Print and shaded views of the part. All mm, measured from the part's lowest x, y and z. Round coordinates to 2 decimals unless told otherwise and drop trailing zeros. Write each loop counter-clockwise with the first axis right and the second up, starting at its lowest first coordinate (ties: lowest second). Pieces come first, ordered by that corner, then holes. Notation, with made-up numbers: (58.5, 55.5) - (73.5, 55.5) arc R29 ccw to (73.5, 93.5) - close; hole circle Ø6 at (81, 75.25). An arc over 180 degrees is marked (long way). Put each result on its own line as item: value. Start each with the question number.
Item 1: Cut at A-A (x = 15.24). Give the cut face in (y, z) (1 decimal).
Item 2: Pin check, flat tips, straight feed: pin 1 Ø5 at (y, z) = (7.5, 146) entering from +X; pin 2 Ø1.5 at (x, z) = (104, 76.5) entering from +Y (3 decimals); pin 3 Ø3.5 at (x, y) = (124.26, 9.325) entering from -Z; pin 4 Ø5.5 at (x, y) = (69.75, 9.325) entering from -Z. Stop position of each tip, or through.
Item 3: Cut at B-B (z = 50). Give the cut face in (x, y) (1 decimal), and give its area (3 significant figures).
Item 4: Cut at C-C (x = 51.5). Give the cut face in (y, z) (1 decimal).
Item 5: Drill centre lines: line 1 (X direction, y = 9, z = 141); line 2 (Y direction, x = 57.5, z = 35.5) (1 decimal); line 3 (X direction, y = 4.25, z = 141.5). Where is each one in solid material? Low to high. Write a range as from..to.
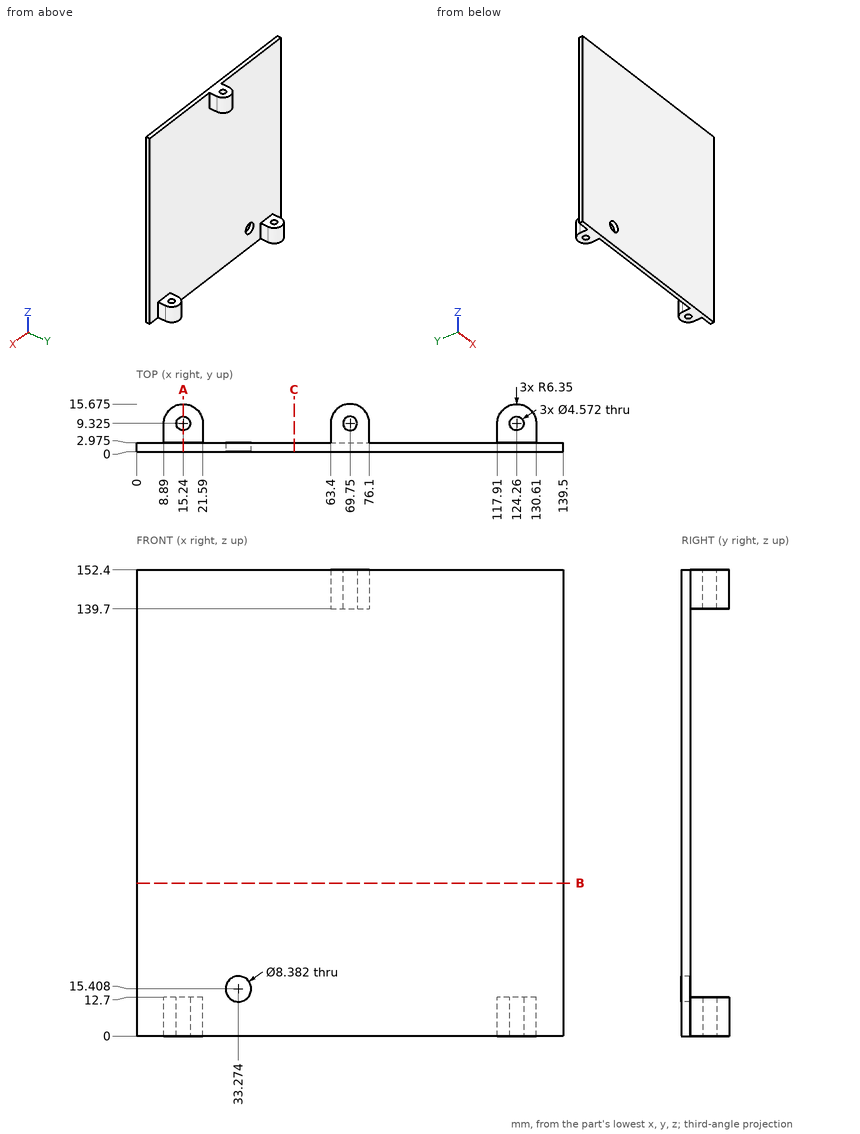
Output values:
1. outline: (0, 0) - (7, 0) - (7, 12.7) - (3, 12.7) - (3, 152.4) - (0, 152.4) - close; (11.6, 0) - (15.7, 0) - (15.7, 12.7) - (11.6, 12.7) - close
2. pin 1: x = 76.1
2. pin 2: y = 2.975
2. pin 3: through
2. pin 4: z = 139.7
3. outline: (0, 0) - (139.5, 0) - (139.5, 3) - (0, 3) - close
3. area: 415 mm2
4. outline: (0, 0) - (3, 0) - (3, 152.4) - (0, 152.4) - close
5. line 1: 63.4..67.49, 72.01..76.1
5. line 2: 0..3
5. line 3: 63.4..76.1
